Autodesk Inventor part; units mm, degrees
ref_plane "YZ Plane" through (0, 0, 0) normal (1, 0, 0) x (0, 1, 0)
ref_plane "XZ Plane" through (0, 0, 0) normal (0, 1, 0) x (-1, 0, 0)
ref_plane "XY Plane" through (0, 0, 0) normal (0, 0, 1) x (1, 0, 0)
sketch "Эскиз1" plane through (0, 0, 0) normal (0, 1, 0) x (-1, 0, 0)
  line L0 (3.1376, 6.642) -> (-6.8624, 6.642)
  line L1 (-6.8624, 6.642) -> (-6.8624, 3.642)
  line L2 (3.1376, 6.642) -> (3.1376, 3.642)
  line L3 (3.1376, 3.642) -> (2.077, 2.5813)
  line L4 (-6.8624, 3.642) -> (-5.8017, 2.5813)
  line L5 (2.077, 2.5813) -> (2.077, -4.4187)
  line L6 (2.077, -4.4187) -> (1.3699, -5.1258)
  line L7 (-5.8017, 2.5813) -> (-5.8017, -4.4187)
  line L8 (-5.8017, -4.4187) -> (-5.0946, -5.1258)
  line L9 (1.3699, -5.1258) -> (-5.0946, -5.1258)
  line L10 (-1.8624, 6.642) -> (-1.8624, -5.1258)
  point P0 (0, 0)
revolve "Вращение1" add sketch "Эскиз1" angle 360 about axis through (1.8624, 0, 6.642) along (0, 0, -1) contours L2 L3 L5 L6 L9 L10 L0
sketch "Эскиз6" plane through (1.8624, 0, 6.642) normal (0, 0, 1) x (1, 0, 0)
  circle A0 centre (0, 0) radius 3.2322
  circle A1 centre (-2.5, 0) radius 1
  circle A2 centre (2.5, 0) radius 1
sketch3d "3D эскиз3"
  line L0 (-0.6376, 0, 6.642) -> (-0.6376, 0, 12.642)
sweep "Сдвиг2" add profiles "Эскиз6" path "3D эскиз3" contours A0 A2 | A0 A2 | A1 A0 | A0 A1
CAD build for the part. Positions are in the model's coordinates, mm. A direction names the side the tool comes from. Round coordinates to 2 decimals unless told otherwise and drop trailing zeros. Order: outer loops, then holes, each group sorted by start corner. A loop starts at its lowest first (then second) coordinate and runs counter-clockwise, first axis right, second up. Notation, with made-up numbers: (-24, -15) - (32, -15) arc R16 ccw to (32, 11) - close; hole circle Ø8 at (87, 8.25). An arc over 180 degrees is marked (long way). Answer in a Markdown table with one row per item. Add a question column.
(1) Drop flat-ended pins along their axis: pin 1 Ø6 at (x, y) = (-1.5, 1.5) entering from +Z; pin 2 Ø3 at (y, z) = (-3, 1.5) entering from +X; pin 3 Ø3 at (x, z) = (-1, 10) entering from -Y; pin 4 Ø5 at (y, z) = (0, 0) entering from +X. Give the stop position or say it passes through.
(2) 3-axis set-ups, long thin cutter, end or side, ignore diameter. For faces 1 (the face through (6.858, 0.22, 5.121)), 2 (the face through (5.286, -0.383, 9.684)): which of +Z, -Z, +X, -X, +Y, -Y reach the whole face in a straight line?
(3) Probe L1, parallel to Z at x = 3, y = -1.25; L2, parallel to X at y = -0.25, z = 7.5; L3, parallel to X at y = -3, z = -2.75. List the from-to ranges inside material, lowest first. Write a range as [from, to].
(4) Band-saw the part on D-D on z = 6. List the corners of the cut face in (x, y).
(5) Mould opens along X. For faces 3 (the face through (4, 0, 12.642)), 4 (the face through (2.375, 3.906, -0.968)), 5 (the face through (-0.2, -0.9, 9.7)) say: +X half, -X half, draft (parallel to the pull), parting line (faces both ways), or undercut.
(6) Band-saw the part on B-B on z = 8.5. List the corners of the cut face in (x, y).
(7) Band-saw the part on A-A on y = 0. List the corners of the cut face in (x, z).
(8) Band-saw the part on C-C on z = 2. List the corners of the cut face in (x, y), and give its area (3 significant figures).
Data:
| question | item | result |
|---|---|---|
| 1 | pin 1 | stops at z = 12.64 |
| 1 | pin 2 | stops at x = 5.51 |
| 1 | pin 3 | stops at y = -1 |
| 1 | pin 4 | stops at x = 5.8 |
| 2 | face 1 | +Z, -Z |
| 2 | face 2 | +Z |
| 3 | L1 | z = [-5.13, 6.64] |
| 3 | L2 | x = [-1.61, 0.33], [3.39, 5.33] |
| 3 | L3 | x = [-0.69, 4.42] |
| 4 | outline | circle Ø10 at (1.86, 0) |
| 5 | face 3 | draft |
| 5 | face 4 | parting line |
| 5 | face 5 | undercut |
| 6 | outline | circle Ø2 at (-0.64, 0); circle Ø2 at (4.36, 0) |
| 7 | outline | (-3.14, 3.64) - (-2.08, 2.58) - (-2.08, -4.42) - (-1.37, -5.13) - (5.09, -5.13) - (5.8, -4.42) - (5.8, 2.58) - (6.86, 3.64) - (6.86, 6.64) - (5.36, 6.64) - (5.36, 12.64) - (3.36, 12.64) - (3.36, 6.64) - (0.36, 6.64) - (0.36, 12.64) - (-1.64, 12.64) - (-1.64, 6.64) - (-3.14, 6.64) - close |
| 8 | outline | circle Ø7.88 at (1.86, 0) |
| 8 | area | 48.8 mm^2 |
